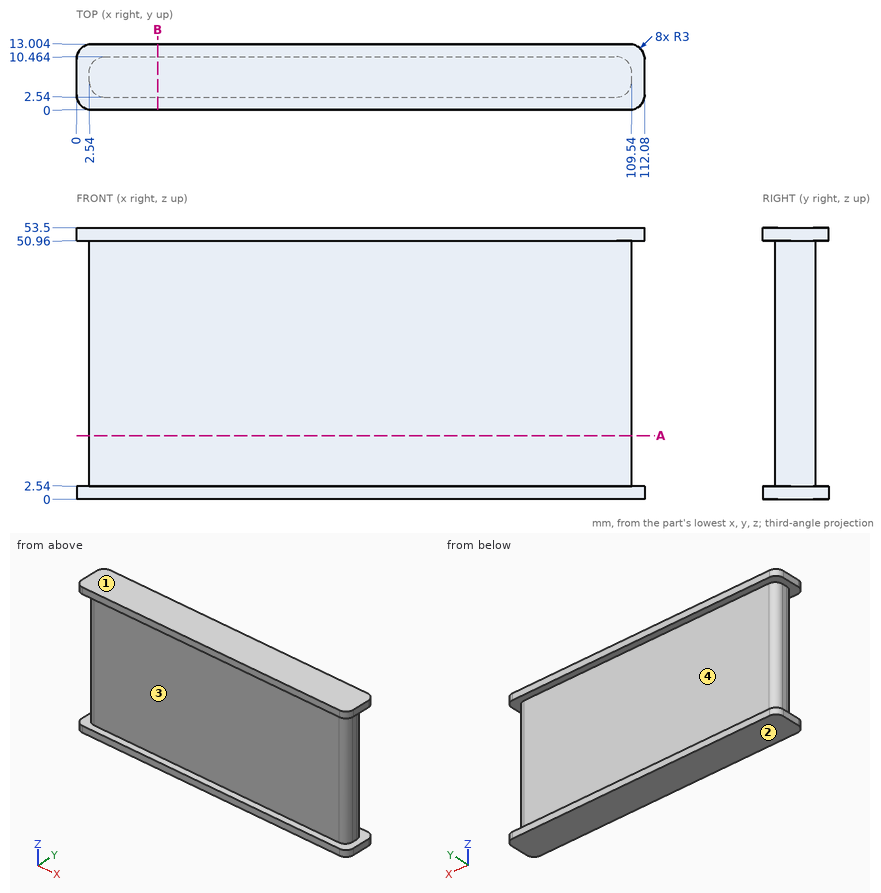
Part print with two shaded views. Sizes in mm from the minimum x, y, z corner. Round coordinates to 2 decimals unless told otherwise and drop trailing zeros. Order: outer loops, then holes, each group sorted by start corner. A loop starts at its lowest first (then second) coordinate and runs counter-clockwise, first axis right, second up. Notation, with made-up numbers: M 29,-21.5 L 33,-21.5 A11 ccw 33,-12.5 Z; hole C 15.5,-40 d6. An arc over 180 degrees is marked long. Put each result on its own line as item: value. Start each with the question number.
1. Drill centre lines: probe 1 along Z at (x, y) = (69, 12.75); probe 2 along Y at (x, z) = (102, 49); probe 3 along X at (y, z) = (5.5, 8). Where is each one in solid material? Low to high. Write a range as [from, to].
2. Drop flat-ended pins along their axis: pin 1 (2 mm diameter, centred on y = 6.5, z = 20.5, fed in from +X); pin 2 (1 mm diameter, centred on x = 86.5, z = 30.5, fed in from +Y); pin 3 (1.5 mm diameter, centred on y = 7, z = 20, fed in from -X). Give the stop position or say it passes through.
3. Slice it at A-A on z = 12.5. List the corners of the cut face in (x, y), then the cut area to 3 significant figures.
4. Slice it at B-B on x = 16. List the corners of the cut face in (y, z).
5. Two-plate mould, pull along Z, no slides. Class the marked faces 1, 2, 3 and 4: +Z half, -Z half, draft (parallel to the pull), parting line (faces both ways), or undercut.
Findings:
1. probe 1: [0, 2.54], [50.96, 53.5]
1. probe 2: [2.54, 10.46]
1. probe 3: [2.54, 109.54]
2. pin 1: x = 109.54
2. pin 2: y = 10.46
2. pin 3: x = 2.54
3. outline: M 2.54,5.54 A3 ccw 5.54,2.54 L 106.54,2.54 A3 ccw 109.54,5.54 L 109.54,7.46 A3 ccw 106.54,10.46 L 5.54,10.46 A3 ccw 2.54,7.46 Z
3. area: 840 mm2
4. outline: M 0,0 L 13,0 L 13,2.54 L 10.46,2.54 L 10.46,50.96 L 13,50.96 L 13,53.5 L 0,53.5 L 0,50.96 L 2.54,50.96 L 2.54,2.54 L 0,2.54 Z
5. face 1: +Z half
5. face 2: -Z half
5. face 3: undercut
5. face 4: undercut
